from build123d import *

# Parameters (mm, degrees)
BOSS_EXTRUDE2_DEPTH = 3


with BuildPart() as part:
    # Sketch1 → Boss-Extrude2 (new body)
    with BuildSketch(Plane.XY):
        with BuildLine():
            ThreePointArc((-24.781290204, -3.3929583), (-28.4, 0), (-24.781290204, 3.3929583))
            Line((-24.781290204, 3.3929583), (-12.188441083, 2.581224344))
            ThreePointArc((-12.188441083, 2.581224344), (-14.492522891, 7.771208774), (-18.780288742, 11.494083385))
            add(Edge.make_bspline(
                [(-25, 13.069), (-21.982355601, 12.146946089), (-18.780288742, 11.494083385)],
                knots=[0, 0, 0, 0.145973682, 0.145973682, 0.145973682], degree=2))
            ThreePointArc((-25, 13.069), (-38.069, 0), (-25, -13.069))
            add(Edge.make_bspline(
                [(-25, -13.069), (-21.982355601, -12.146946089), (-18.780288742, -11.494083385)],
                knots=[0, 0, 0, 0.145973682, 0.145973682, 0.145973682], degree=2))
            ThreePointArc((-18.780288742, -11.494083385), (-14.492522891, -7.771208774), (-12.188441083, -2.581224344))
            Line((-12.188441083, -2.581224344), (-24.781290204, -3.3929583))
        make_face()
        with BuildLine():
            ThreePointArc((-18.780288742, 11.494083385), (-14.492522891, 7.771208774), (-12.188441083, 2.581224344))
            Line((-12.188441083, 2.581224344), (-3.107347179, 1.995857823))
            ThreePointArc((-3.107347179, 1.995857823), (-1.236, 0), (-3.107347179, -1.995857823))
            Line((-3.107347179, -1.995857823), (-12.188441083, -2.581224344))
            ThreePointArc((-12.188441083, -2.581224344), (-14.492522891, -7.771208774), (-18.780288742, -11.494083385))
            add(Edge.make_bspline(
                [(-18.780288742, -11.494083385), (-1.944343038, -8.061437688), (19.989933944, -12.070542619)],
                knots=[0.145973682, 0.145973682, 0.145973682, 0.91347951, 0.91347951, 0.91347951], degree=2))
            ThreePointArc((19.989933944, -12.070542619), (14.904735293, -8.299662132), (12.188441083, -2.581224344))
            Line((12.188441083, -2.581224344), (3.107347179, -1.995857823))
            ThreePointArc((3.107347179, -1.995857823), (1.236, 0), (3.107347179, 1.995857823))
            Line((3.107347179, 1.995857823), (12.188441083, 2.581224344))
            ThreePointArc((12.188441083, 2.581224344), (14.904735293, 8.299662132), (19.989933944, 12.070542619))
            add(Edge.make_bspline(
                [(-18.780288742, 11.494083385), (-1.944343038, 8.061437688), (19.989933944, 12.070542619)],
                knots=[0.145973682, 0.145973682, 0.145973682, 0.91347951, 0.91347951, 0.91347951], degree=2))
        make_face()
        with BuildLine():
            add(Edge.make_bspline(
                [(19.989933944, 12.070542619), (22.462572371, 12.522486712), (25, 13.069)],
                knots=[0.91347951, 0.91347951, 0.91347951, 1, 1, 1], degree=2))
            ThreePointArc((19.989933944, 12.070542619), (14.904735293, 8.299662132), (12.188441083, 2.581224344))
            Line((12.188441083, 2.581224344), (24.781290204, 3.3929583))
            ThreePointArc((24.781290204, 3.3929583), (28.4, 0), (24.781290204, -3.3929583))
            Line((24.781290204, -3.3929583), (12.188441083, -2.581224344))
            ThreePointArc((12.188441083, -2.581224344), (14.904735293, -8.299662132), (19.989933944, -12.070542619))
            add(Edge.make_bspline(
                [(19.989933944, -12.070542619), (22.462572371, -12.522486712), (25, -13.069)],
                knots=[0.91347951, 0.91347951, 0.91347951, 1, 1, 1], degree=2))
            ThreePointArc((25, -13.069), (34.241178523, -9.241178523), (38.069, 0))
            ThreePointArc((38.069, 0), (34.241178523, 9.241178523), (25, 13.069))
        make_face()
    extrude(amount=BOSS_EXTRUDE2_DEPTH)


solid = part.part
Here's how the part is built. I have some questions about the finished solid (model axes, mm). A direction names the side the tool comes from. Give positions to 0.01 mm unless a question says otherwise; leave off trailing zeros. Order: outer loops, then holes, each group sorted by start corner. A loop starts at its lowest first (then second) coordinate and runs counter-clockwise, first axis right, second up. Notation, with made-up numbers: M 74.5,62 L 103.5,62 A26 cw 103.5,76 Z; hole C -15.75,-4 d7. An arc over 180 degrees is marked long. Answer as a JSON object with one key per item and string values. Group by question number.
1) Suppose I cut it at C-C, the plane x = -31. Write out the boundary of the cut face in (y, z), plus the area to 3 significant figures.
2) Suppose I cut it at B-B, the plane y = 6.5. Write out the boundary of the cut face in (x, z).
3) Please list where these lines run through material, in increasing order: L1, parallel to X at y = 1.25, z = 2.4; L2, parallel to X at y = -1, z = 2.8; L3, parallel to Y at x = -10.5, z = 1.5. Write a range as [from, to].
4) I'm going to push flat-ended pins straight in: pin 1 Ø1.5 at (x, z) = (-4, 1.5) entering from +Y; pin 2 Ø1 at (x, z) = (14, 1.5) entering from +Y; pin 3 Ø1 at (y, z) = (-5, 0.5) entering from +X. Where does each tip first touch, or does it pass through?
5) We'd pull the mould along Y, two halves only. Please class faces 1 (the cylindrical face through (-28.4, -0.1, 1.5)), 2 (the cylindrical face through (-38.066, 0.287, 1.479)), 3 (the cylindrical face through (28.4, 0.1, 1.5)), 4 (the flat face through (-1, 0, 3)): pulls with the +Y half, pulls with the -Y half, needs draft (parallel to the pull), parting line crosses it, or undercut.
6) On a 3-axis mill with a long thin cutter (end or side, diameter ignored), from which of +Z, -Z, +X, -X, +Y, -Y can I reach the whole of each face in a straight line? I mean faces 5 (the flat face through (-1, 0, 0)), 6 (the flat face through (-14.096, 2.704, 1.479)). Say none if no direction works.
7) Suppose I cut it at A-A, the plane z = 0.95. Count the separate pieces of the cut face and the enclosed holes in it, plus the area to 3 significant figures.
Results found:
{
 "1": {"outline": "M -11.61,0 L 11.61,0 L 11.61,3 L -11.61,3 Z", "area": "69.7 mm²"},
 "2": {"outline": "M -36.34,0 L 36.34,0 L 36.34,3 L -36.34,3 Z"},
 "3": {"L1": "[-38.01, -28.16], [-1.67, 1.67], [28.16, 38.01]", "L2": "[-38.03, -28.25], [-1.5, 1.5], [28.25, 38.03]", "L3": "[-10.28, -2.47], [2.47, 10.28]"},
 "4": {"pin 1": "y = 9.95", "pin 2": "y = 11.17", "pin 3": "x = 37.27"},
 "5": {"face 1": "undercut", "face 2": "parting line crosses it", "face 3": "undercut", "face 4": "needs draft"},
 "6": {"face 5": "-Z, +X, -X, +Y, -Y", "face 6": "+Z, -Z"},
 "7": {"separate pieces": "1", "enclosed holes": "2", "area": "1,350 mm²"}
}
